from build123d import *

# Parameters (mm, degrees)
SKETCH1_W            = 177.8
SKETCH1_H            = 177.8
BOSS_EXTRUDE1_DEPTH  = 152.4
SKETCH2_W            = 127
SKETCH2_H            = 106.68
CUT_EXTRUDE1_DEPTH   = 152.4
SKETCH3_R            = 19.05
CUT_EXTRUDE2_DEPTH   = 182.626
SKETCH4_W            = 152.4
SKETCH4_H            = 71.12
BOSS_EXTRUDE2_DEPTH  = 825.5
SKETCH5_W            = 152.4
SKETCH5_H            = 71.12
BOSS_EXTRUDE3_DEPTH  = 825.5
SKETCH6_W            = 76.2
SKETCH6_H            = 152.4
BOSS_EXTRUDE4_DEPTH  = 457.2
SKETCH7_W            = 101.6
SKETCH7_H            = 50.8
BOSS_EXTRUDE9_DEPTH  = 50.8
SKETCH12_W           = 101.6
SKETCH12_H           = 50.8
BOSS_EXTRUDE10_DEPTH = 50.8
SKETCH13_W           = 101.6
SKETCH13_H           = 50.8
BOSS_EXTRUDE11_DEPTH = 50.8
SKETCH14_W           = 101.6
SKETCH14_H           = 50.8
BOSS_EXTRUDE12_DEPTH = 50.8
SKETCH15_W           = 50.8
SKETCH15_H           = 101.6
BOSS_EXTRUDE13_DEPTH = 76.2
SKETCH16_W           = 50.8
SKETCH16_H           = 101.6
BOSS_EXTRUDE14_DEPTH = 76.2
SKETCH17_R           = 6.35
CUT_EXTRUDE3_DEPTH   = 205.994
SKETCH18_R           = 6.35
CUT_EXTRUDE4_DEPTH   = 205.994


with BuildPart() as part:
    # Sketch1 → Boss-Extrude1 (new body)
    with BuildSketch(Plane.XY):
        with Locations((88.9, 88.9)):
            Rectangle(SKETCH1_W, SKETCH1_H)
    extrude(amount=BOSS_EXTRUDE1_DEPTH)

    # Sketch2 → Cut-Extrude1 (cut)
    with BuildSketch(Plane.XY.offset(152.4)):
        with Locations((88.9, 53.34)):
            Rectangle(SKETCH2_W, SKETCH2_H)
    extrude(amount=-CUT_EXTRUDE1_DEPTH, mode=Mode.SUBTRACT)

    # Sketch3 → Cut-Extrude2 (cut)
    with BuildSketch(Plane(origin=(177.8, 0, 0), x_dir=(0, 0, -1), z_dir=(1, 0, 0))):
        with Locations((-76.2, 45.72)):
            Circle(SKETCH3_R)
    extrude(amount=-CUT_EXTRUDE2_DEPTH, mode=Mode.SUBTRACT)

    # Sketch4 → Boss-Extrude2 (add)
    with BuildSketch(Plane(origin=(177.8, 0, 0), x_dir=(0, 0, -1), z_dir=(1, 0, 0))):
        with Locations((-76.2, 142.24)):
            Rectangle(SKETCH4_W, SKETCH4_H)
    extrude(amount=BOSS_EXTRUDE2_DEPTH)

    # Sketch5 → Boss-Extrude3 (add)
    with BuildSketch(Plane.ZY):
        with Locations((76.2, 142.24)):
            Rectangle(SKETCH5_W, SKETCH5_H)
    extrude(amount=BOSS_EXTRUDE3_DEPTH)

    # Sketch6 → Boss-Extrude4 (add)
    with BuildSketch(Plane(origin=(0, 177.8, 0), x_dir=(1, 0, 0), z_dir=(0, 1, 0))):
        with Locations((-787.4, -76.2)):
            Rectangle(SKETCH6_W, SKETCH6_H)
        with Locations((965.2, -76.2)):
            Rectangle(SKETCH6_W, SKETCH6_H)
    extrude(amount=BOSS_EXTRUDE4_DEPTH)

    # Sketch7 → Boss-Extrude9 (add)
    with BuildSketch(Plane.ZY.offset(825.5)):
        with Locations((76.2, 609.6)):
            Rectangle(SKETCH7_W, SKETCH7_H)
    extrude(amount=BOSS_EXTRUDE9_DEPTH)

    # Sketch12 → Boss-Extrude10 (add)
    with BuildSketch(Plane(origin=(-749.3, 0, 0), x_dir=(0, 0, -1), z_dir=(1, 0, 0))):
        with Locations((-76.2, 609.6)):
            Rectangle(SKETCH12_W, SKETCH12_H)
    extrude(amount=BOSS_EXTRUDE10_DEPTH)

    # Sketch13 → Boss-Extrude11 (add)
    with BuildSketch(Plane.ZY.offset(-927.1)):
        with Locations((76.2, 609.6)):
            Rectangle(SKETCH13_W, SKETCH13_H)
    extrude(amount=BOSS_EXTRUDE11_DEPTH)

    # Sketch14 → Boss-Extrude12 (add)
    with BuildSketch(Plane(origin=(1003.3, 0, 0), x_dir=(0, 0, -1), z_dir=(1, 0, 0))):
        with Locations((-76.2, 609.6)):
            Rectangle(SKETCH14_W, SKETCH14_H)
    extrude(amount=BOSS_EXTRUDE12_DEPTH)

    # Sketch15 → Boss-Extrude13 (add)
    with BuildSketch(Plane(origin=(0, 635, 0), x_dir=(1, 0, 0), z_dir=(0, 1, 0))):
        with Locations((901.7, -76.2)):
            Rectangle(SKETCH15_W, SKETCH15_H)
        with Locations((1028.7, -76.2)):
            Rectangle(SKETCH15_W, SKETCH15_H)
    extrude(amount=BOSS_EXTRUDE13_DEPTH)

    # Sketch16 → Boss-Extrude14 (add)
    with BuildSketch(Plane(origin=(0, 635, 0), x_dir=(1, 0, 0), z_dir=(0, 1, 0))):
        with Locations((-723.9, -76.2)):
            Rectangle(SKETCH16_W, SKETCH16_H)
        with Locations((-850.9, -76.2)):
            Rectangle(SKETCH16_W, SKETCH16_H)
    extrude(amount=BOSS_EXTRUDE14_DEPTH)

    # Sketch17 → Cut-Extrude3 (cut)
    with BuildSketch(Plane.ZY.offset(876.3)):
        with Locations((76.2, 673.1)):
            Circle(SKETCH17_R)
    extrude(amount=-CUT_EXTRUDE3_DEPTH, mode=Mode.SUBTRACT)

    # Sketch18 → Cut-Extrude4 (cut)
    with BuildSketch(Plane(origin=(1054.1, 0, 0), x_dir=(0, 0, -1), z_dir=(1, 0, 0))):
        with Locations((-76.2, 673.1)):
            Circle(SKETCH18_R)
    extrude(amount=-CUT_EXTRUDE4_DEPTH, mode=Mode.SUBTRACT)


solid = part.part
Source: CAD feature listing. Evaluate the final solid. Frame: model axes, mm. A direction names the side the tool comes from. Give positions to 0.01 mm unless a question says otherwise; leave off trailing zeros. Write each loop counter-clockwise with the first axis right and the second up, starting at its lowest first coordinate (ties: lowest second). Pieces come first, ordered by that corner, then holes. Notation, with made-up numbers: (17.25, 13) -> (64.25, 13) arc R18 ccw to (64.25, 48) -> close; hole circle Ø7 at (-28.5, 80). An arc over 180 degrees is marked (long way). Write item = value, one per line.
Q1. Cut plane C-C on x = -524. Return loops of the section in (y, z).
Here are the results:
outline = (106.68, 0) -> (177.8, 0) -> (177.8, 152.4) -> (106.68, 152.4) -> close
Q2. Cut plane A-A on y = 566. Return loops of the section in (x, z).
Here are the results:
outline = (-825.5, 0) -> (-749.3, 0) -> (-749.3, 152.4) -> (-825.5, 152.4) -> close; (927.1, 0) -> (1003.3, 0) -> (1003.3, 152.4) -> (927.1, 152.4) -> close
Q3. Cut plane B-B on y = 45.72. Return loops of the section in (x, z).
Here are the results:
outline = (0, 0) -> (25.4, 0) -> (25.4, 57.15) -> (0, 57.15) -> close; (0, 95.25) -> (25.4, 95.25) -> (25.4, 152.4) -> (0, 152.4) -> close; (152.4, 0) -> (177.8, 0) -> (177.8, 57.15) -> (152.4, 57.15) -> close; (152.4, 95.25) -> (177.8, 95.25) -> (177.8, 152.4) -> (152.4, 152.4) -> close
Q4. Line query: line 1 (Y direction, x = 899, z = 76.2); line 2 (X direction, y = 348, z = 107); line 3 (Y direction, x = 1027, z = 76.2). Output: solid intervals per line, ascending. Write a range as from..to.
Here are the results:
line_1 = 106.68..177.8, 584.2..666.75, 679.45..711.2
line_2 = -825.5..-749.3, 927.1..1003.3
line_3 = 584.2..666.75, 679.45..711.2
Q5. Mould query, pull axis X, two halves, no side actions, for faces 6 (the face through (-876.3, 649, 75)), 7 (the face through (901, 647, 25.4)), 8 (the face through (177.8, 53, 58)), 9 (the face through (1028, 647, 25.4)). Classes: +X half, -X half, draft (parallel to the pull), parting line (faces both ways), or undercut.
Here are the results:
face_6 = -X half
face_7 = undercut
face_8 = +X half
face_9 = draft
Q6. First-contact query: pin 1 (5 mm diameter, centred on y = 372, z = 134, fed in from +X); pin 2 (4 mm diameter, centred on y = 119.5, z = 40.5, fed in from -X); pin 3 (1.5 mm diameter, centred on x = 132.5, z = 17, fed in from -Y); pin 4 (10 mm diameter, centred on y = 673.1, z = 76.2, fed in from -X) (1 decimal). Flat tips, straight axial feed; report the tip coordinate or a pass-through.
Here are the results:
pin_1 = 1003.3
pin_2 = -825.5
pin_3 = 106.68
pin_4 = through
Q7. Reachability of faces 1 (the face through (1003.3, 664, 77)), 2 (the face through (585, 106.68, 77)), 3 (the face through (902, 584.2, 75)), 4 (the face through (-851, 647, 127)), 5 (the face through (1028, 647, 127)) from +Z, -Z, +X, -X, +Y, -Y: full face, straight path, thin tool, end or side. Return the list, or none.
Here are the results:
face_1 = +Z, -Z, +Y
face_2 = +Z, -Z, +X, -Y
face_3 = +Z, -Z
face_4 = +Z, -X, +Y, -Y
face_5 = +Z, +X, +Y, -Y
